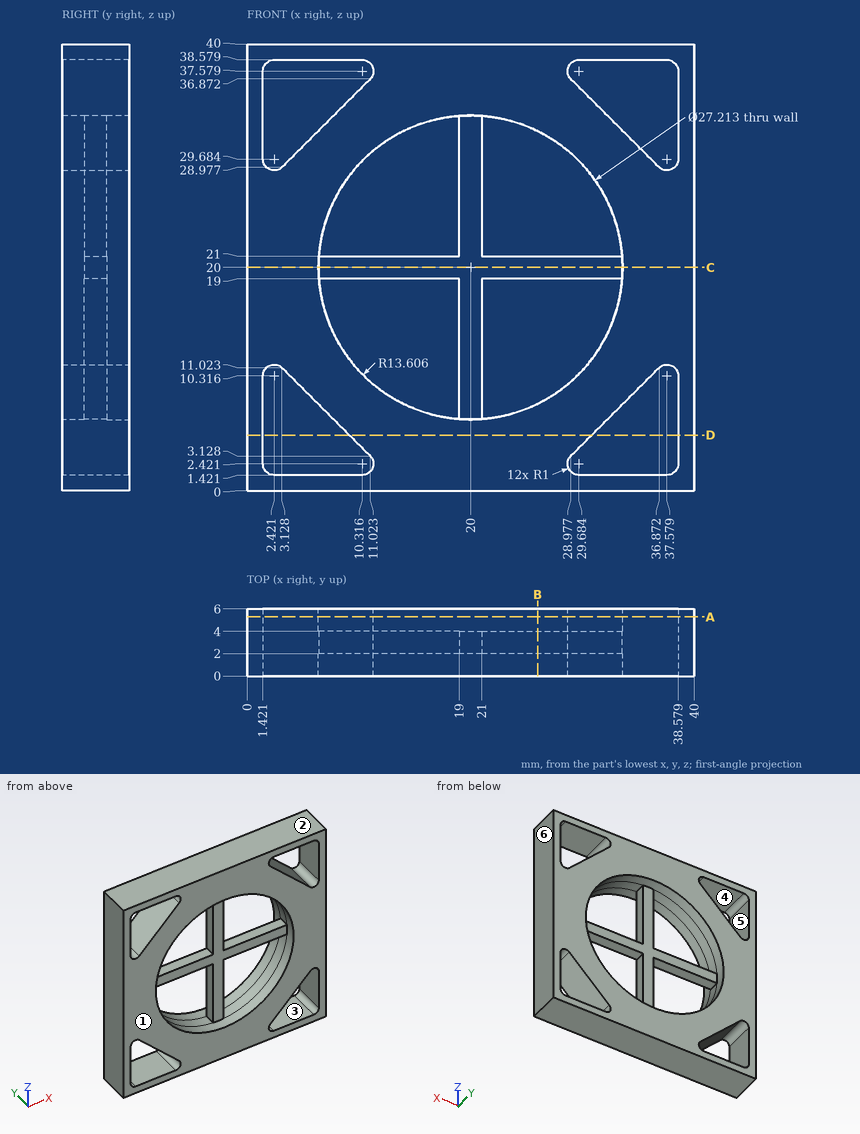
Part print with two shaded views. Sizes in mm from the minimum x, y, z corner. A direction names the side the tool comes from. Round coordinates to 2 decimals unless told otherwise and drop trailing zeros. Order: outer loops, then holes, each group sorted by start corner. A loop starts at its lowest first (then second) coordinate and runs counter-clockwise, first axis right, second up. Notation, with made-up numbers: (6.25, 79) -> (10.25, 79) arc R27 ccw to (10.25, 95) -> close; hole circle Ø5 at (-16.75, 73). An arc over 180 degrees is marked (long way). One line per question, with ' | ' between items.
Q1. Two-plate mould, pull along Z, no slides. Class the marked faces 1, 2, 3 and 4: released by +Z, released by -Z, zero draft, split by the parting line, or undercut.
Completed:
face 1: zero draft | face 2: released by +Z | face 3: undercut | face 4: undercut
Q2. Which spindle directions (+Z, -Z, +X, -X, +Y, -Y) get a long thin tool onto all of the face, cutting with end or side? Do the marked faces 5 and 6. Say none if no direction does.
Completed:
face 5: +Y, -Y | face 6: +Z, -Z, +X, +Y, -Y
Q3. Probe probe 1 along X at (y, z) = (5.5, 20); probe 2 along Z at (x, y) = (36.5, 0.4). List the from-to ranges inside material, lowest first.
Completed:
probe 1: x = 0 to 6.39, 33.61 to 40 | probe 2: z = 0 to 1.42, 10.65 to 29.35, 38.58 to 40
Q4. Slice it at C-C (z = 20). Write the cut outline in (x, y).
Completed:
outline: (0, 0) -> (6.39, 0) -> (6.39, 2) -> (33.61, 2) -> (33.61, 0) -> (40, 0) -> (40, 6) -> (33.61, 6) -> (33.61, 4) -> (6.39, 4) -> (6.39, 6) -> (0, 6) -> close
Q5. Slice it at B-B (x = 26). Write the cut outline in (y, z).
Completed:
outline: (0, 0) -> (6, 0) -> (6, 7.79) -> (0, 7.79) -> close; (0, 32.21) -> (6, 32.21) -> (6, 40) -> (0, 40) -> close; (2, 19) -> (4, 19) -> (4, 21) -> (2, 21) -> close
Q6. Slice it at D-D (z = 5). Write the cut outline in (x, y), then the cut area to 3 significant figures.
Completed:
outline: (0, 0) -> (1.42, 0) -> (1.42, 6) -> (0, 6) -> close; (9.15, 0) -> (30.85, 0) -> (30.85, 6) -> (9.15, 6) -> close; (38.58, 0) -> (40, 0) -> (40, 6) -> (38.58, 6) -> close | area: 147 mm^2
Q7. Drop a flat-ended pin along its axis: pin 1 (10 mm diameter, centred on x = 28, z = 18, fed in from -Y). Give the stop position or say it passes through.
Completed:
pin 1: stops at y = 2
Q8. Slice it at A-A (y = 5.3). Give the number of separate pieces and of enclosed holes in the cut face.
Completed:
separate pieces: 1 | enclosed holes: 5
